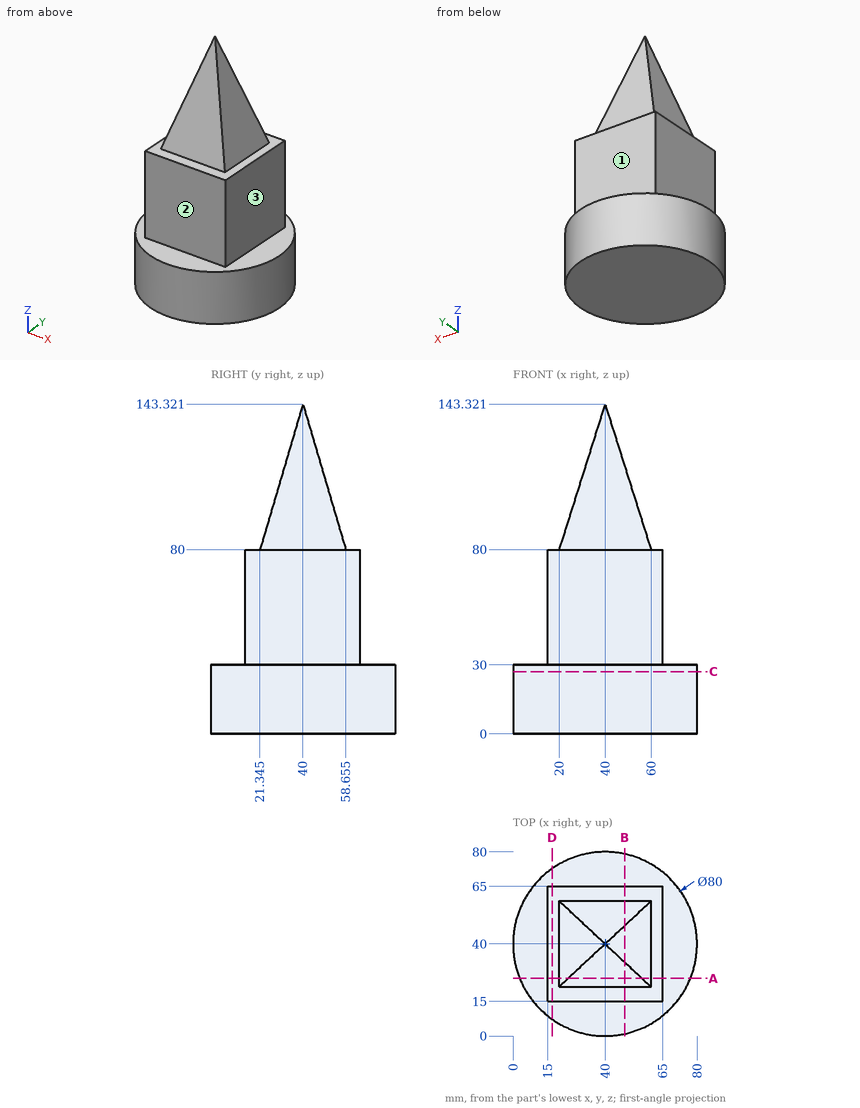
Here's the drawing with two shaded views (mm, measured from the low corner). I have some questions. A direction names the side the tool comes from. Coordinates: 2 decimals unless noted, no trailing zeros. Loops run counter-clockwise (first coordinate to the right, second up) from the corner with the lowest first, then second, coordinate; pieces in that order, holes last. Notation, with made-up numbers: M -11.5,87 L 12.5,87 A25 ccw 12.5,119 Z; hole C 78,49 d4. An arc over 180 degrees is marked long. Return JSON: item names as keys, results as strings. Group by question number.
Item 1: Imagine slicing it at D-D (x = 17). Please give me the cut outline in (y, z), and give its area (3 significant figures).
Item 2: Imagine slicing it at B-B (x = 48.5). Please give me the cut outline in (y, z) (1 decimal), and give its area (3 significant figures).
Item 3: I'm going to push flat-ended pins straight in: pin 1 Ø1 at (x, z) = (13.5, 44) entering from +Y; pin 2 Ø1 at (x, z) = (64.5, 46.5) entering from -Y; pin 3 Ø5 at (y, z) = (32, 15.5) entering from +X; pin 4 Ø25 at (y, z) = (36.5, 61.5) entering from +X. Where does each tip first touch, or does it pass through?
Item 4: Imagine slicing it at A-A (y = 25). Please give me the cut outline in (x, z), and give its area (3 significant figures).
Item 5: On a 3-axis mill with a long thin cutter (end or side, diameter ignored), from which of +Z, -Z, +X, -X, +Y, -Y can I reach the whole of each face in a straight line? I mean the marked faces 1, 2 and 3. Say none if no direction works.
Item 6: If I drill on L1, parallel to Z at x = 42, y = 61.5; L2, parallel to Y at x = 18.5, z = 39.5; L3, parallel to X at y = 41, z = 14, over which ranges is the centre line in solid material (lowest first)? Write a range as from..to.
Item 7: Imagine slicing it at C-C (z = 27). Please give me the cut outline in (x, y), and give its area (3 significant figures).
Verdict:
{
 "1": {"outline": "M 7.27,0 L 72.73,0 L 72.73,30 L 65,30 L 65,80 L 15,80 L 15,30 L 7.27,30 Z", "area": "4,460 mm^2"},
 "2": {"outline": "M 0.9,0 L 79.1,0 L 79.1,30 L 65,30 L 65,80 L 58.7,80 L 47.9,116.4 L 32.1,116.4 L 21.3,80 L 15,80 L 15,30 L 0.9,30 Z", "area": "5,810 mm^2"},
 "3": {"pin 1": "passes through", "pin 2": "stops at y = 15", "pin 3": "stops at x = 79.62", "pin 4": "stops at x = 65"},
 "4": {"outline": "M 2.92,0 L 77.08,0 L 77.08,30 L 65,30 L 65,80 L 60,80 L 56.08,92.41 L 23.92,92.41 L 20,80 L 15,80 L 15,30 L 2.92,30 Z", "area": "5,170 mm^2"},
 "5": {"face 1": "+Z, +X, -X, +Y", "face 2": "+Z, +X, -X, -Y", "face 3": "+Z, +X, +Y, -Y"},
 "6": {"L1": "z = 0..80", "L2": "y = 15..65", "L3": "x = 0.01..79.99"},
 "7": {"outline": "C 40,40 d80", "area": "5,030 mm^2"}
}
